Here's how the part is built. I have some questions about the finished solid (model axes, mm). A direction names the side the tool comes from. Give positions to 0.01 mm unless a question says otherwise; leave off trailing zeros. Loops run counter-clockwise (first coordinate to the right, second up) from the corner with the lowest first, then second, coordinate; pieces in that order, holes last. Notation, with made-up numbers: (28.25, -15.5) - (71.25, -15.5) arc R23 ccw to (71.25, 22.5) - close; hole circle Ø9 at (-39.75, 0). An arc over 180 degrees is marked (long way). One line per item, written item: value. Start each with the question number.
```python
from build123d import *

# Parameters (mm, degrees)
SKETCH1_W           = 76
SKETCH1_H           = 66
SKETCH1_W_2         = 70
SKETCH1_H_2         = 60
BOSS_EXTRUDE1_DEPTH = 18.5
SKETCH2_W           = 76
SKETCH2_H           = 66
SKETCH2_W_2         = 70
SKETCH2_H_2         = 60
BOSS_EXTRUDE2_DEPTH = 27.65
SKETCH4_W           = 76
SKETCH4_H           = 66
BOSS_EXTRUDE3_DEPTH = 10
SKETCH5_R           = 22.6
SKETCH5_R_2         = 19.6
BOSS_EXTRUDE4_DEPTH = 40
FILLET1_R           = 2
FILLET2_R           = 2


with BuildPart() as part:
    # Sketch1 → Boss-Extrude1 (new body)
    with BuildSketch(Plane(origin=(0, 0, 0), x_dir=(1, 0, 0), z_dir=(0, 1, 0))):
        Rectangle(SKETCH1_W, SKETCH1_H)
        Rectangle(SKETCH1_W_2, SKETCH1_H_2, mode=Mode.SUBTRACT)
    extrude(amount=BOSS_EXTRUDE1_DEPTH)

    # Sketch2 → Boss-Extrude2 (add)
    # profile 1 of 2: a face of its own
    with BuildSketch(Plane.XZ):
        Rectangle(SKETCH2_W, SKETCH2_H)
        Rectangle(SKETCH2_W_2, SKETCH2_H_2, mode=Mode.SUBTRACT)
    # profile 2 of 2: a face of its own
    with BuildSketch(Plane.XZ):
        Polygon((-28.95, 10), (-5.225, 10), (-5.225, 30), (-35, 30), (-35, -30), (35, -30), (35, -5), (18.5, -5), (18.5, -10), (-28.95, -10), align=None)
    extrude(amount=BOSS_EXTRUDE2_DEPTH)

    # Sketch4 → Boss-Extrude3 (add)
    with BuildSketch(Plane.XZ.offset(27.65)):
        Rectangle(SKETCH4_W, SKETCH4_H)
    extrude(amount=BOSS_EXTRUDE3_DEPTH)

    # Sketch5 → Boss-Extrude4 (add)
    with BuildSketch(Plane.XZ.offset(37.65)):
        with Locations(Location((0, 0, 0), (0, 0, 270))):
            Circle(SKETCH5_R)
        with Locations(Location((0, 0, 0), (0, 0, 270))):
            Circle(SKETCH5_R_2, mode=Mode.SUBTRACT)
    extrude(amount=BOSS_EXTRUDE4_DEPTH)

    # Fillet1
    fillet1_edges = [part.edges().sort_by_distance(p)[0] for p in [
        (38, -9.575, 33),
        (-38, -9.575, 33),
        (-38, -9.575, -33),
        (38, -9.575, -33),
    ]]
    fillet(fillet1_edges, radius=FILLET1_R)

    # Fillet2
    fillet2_edges = [part.edges().sort_by_distance(p)[0] for p in [
        (0, -37.65, -33),
        (38, -37.65, 0),
        (0, -37.65, 33),
        (-38, -37.65, 0),
        (-37.414213562, -37.65, 32.414213562),
        (37.414213562, -37.65, 32.414213562),
        (-37.414213562, -37.65, -32.414213562),
        (37.414213562, -37.65, -32.414213562),
    ]]
    fillet(fillet2_edges, radius=FILLET2_R)


solid = part.part
```
(1) Please list where these lines run through material, in increasing order: probe 1 along Z at (x, y) = (17.5, -9); probe 2 along X at (y, z) = (-45.5, 0); probe 3 along Z at (x, y) = (29, -26). Write a range as from..to.
(2) If we section it at B-B on z = -25.5: List the corners of the cut face in (x, y) for me.
(3) Will these pins go through, and if not, where does the flat tip stop? pin 1 (5 mm diameter, centred on x = -12.5, z = 8, fed in from +Y); pin 2 (20 mm diameter, centred on x = 15, z = 15, fed in from +Y); pin 3 (12 mm diameter, centred on x = -8, z = -7.5, fed in from -Y).
(4) If we mould it in two halves opening along X, with no side actions, what happens to faces 1 (the face through (7, 1, 30)), 2 (the face through (-38, -8, 0)), 3 (the face through (-1, -8, 33))? For each: pulls with the +X half, pulls with the -X half, needs draft (parallel to the pull), parting line crosses it, or undercut.
(5) If we section it at C-C on x = 0: List the corners of the cut face in (y, z) for me.
(6) If we section it at A-A on y = -18: List the corners of the cut face in (x, z) for me (3 decimals).
(7) If we section it at D-D on y = 7.5: List the corners of the cut face in (x, z) for me.
(8) For faces 4 (the face through (27, -14, -5)), 5 (the face through (-13.8, -57.4, 17.9)), 6 (the face through (-1, -8, -33)), which set-ups out of +Z, -Z, +X, -X, +Y, -Y let a thin tool reach every point of the face, with its end or its side?
Found:
1. probe 1: -33..-10, 30..33
1. probe 2: -22.6..-19.6, 19.6..22.6
1. probe 3: -33..-5, 30..33
2. outline: (-38, -35.65) arc R2 ccw to (-36, -37.65) - (36, -37.65) arc R2 ccw to (38, -35.65) - (38, 18.5) - (35, 18.5) - (35, 0) - (-35, 0) - (-35, 18.5) - (-38, 18.5) - close
3. pin 1: y = 0
3. pin 2: y = -27.65
3. pin 3: y = -37.65
4. face 1: undercut
4. face 2: pulls with the -X half
4. face 3: needs draft
5. outline: (-77.65, -22.6) - (-37.65, -22.6) - (-37.65, -31) arc R2 ccw to (-35.65, -33) - (18.5, -33) - (18.5, -30) - (0, -30) - (0, -10) - (-27.65, -10) - (-27.65, 30) - (18.5, 30) - (18.5, 33) - (-35.65, 33) arc R2 ccw to (-37.65, 31) - (-37.65, 22.6) - (-77.65, 22.6) - (-77.65, 19.6) - (-37.65, 19.6) - (-37.65, -19.6) - (-77.65, -19.6) - close
6. outline: (-38, -31) arc R2 ccw to (-36, -33) - (36, -33) arc R2 ccw to (38, -31) - (38, 31) arc R2 ccw to (36, 33) - (-36, 33) arc R2 ccw to (-38, 31) - close; hole (-28.95, -10) - (18.5, -10) - (18.5, -5) - (35, -5) - (35, 30) - (-5.225, 30) - (-5.225, 10) - (-28.95, 10) - close
7. outline: (-38, -31) arc R2 ccw to (-36, -33) - (36, -33) arc R2 ccw to (38, -31) - (38, 31) arc R2 ccw to (36, 33) - (-36, 33) arc R2 ccw to (-38, 31) - close; hole (-35, -30) - (35, -30) - (35, 30) - (-35, 30) - close
8. face 4: +Y
8. face 5: -Y
8. face 6: -Z, +X, -X, +Y, -Y
